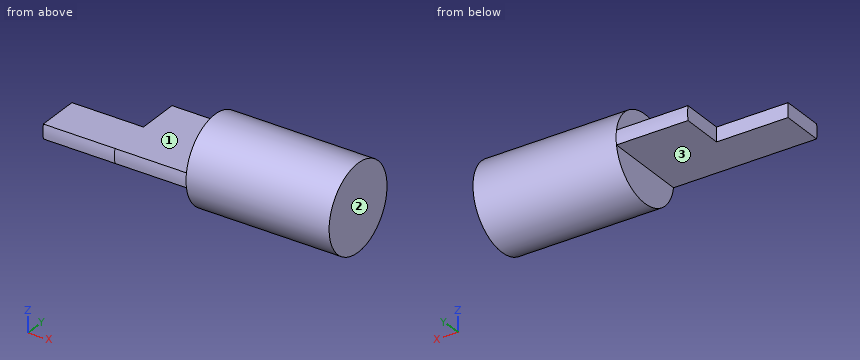
from build123d import *
from build123d.topology import SkipClean

# Parameters (mm, degrees)
SKETCH1_R           = 30
BOSS_EXTRUDE1_DEPTH = 100
BOSS_EXTRUDE2_START = 50
BOSS_EXTRUDE2_DEPTH = 50
BOSS_EXTRUDE3_START = 50
BOSS_EXTRUDE3_DEPTH = 50


with BuildPart() as part:
    # Sketch1 → Boss-Extrude1 (new body)
    with BuildSketch(Plane(origin=(0, 0, 0), x_dir=(0, 0, -1), z_dir=(1, 0, 0))):
        Circle(SKETCH1_R)
    extrude(amount=BOSS_EXTRUDE1_DEPTH)

    # Sketch2 → Boss-Extrude2 (add)
    with SkipClean():  # the faces are left unmerged after this step: merging them gives an invalid solid
        with BuildSketch(Plane.ZY.offset(BOSS_EXTRUDE2_START)):
            with BuildLine():
                Line((5, -29.580398915), (5, 29.580398915))
                ThreePointArc((5, 29.580398915), (0, 30), (-5, 29.580398915))
                Line((-5, 29.580398915), (-5, -29.580398915))
                ThreePointArc((-5, -29.580398915), (0, -30), (5, -29.580398915))
            make_face()
        extrude(amount=-BOSS_EXTRUDE2_DEPTH)

    # Sketch3 → Boss-Extrude3 (add)
    with SkipClean():  # the faces are left unmerged after this step: merging them gives an invalid solid
        with BuildSketch(Plane.ZY.offset(50).offset(BOSS_EXTRUDE3_START)):
            with BuildLine():
                Line((5, 0), (-5, 0))
                Line((-5, 0), (-5, -29.580398915))
                ThreePointArc((-5, -29.580398915), (0, -30), (5, -29.580398915))
                Line((5, -29.580398915), (5, 0))
            make_face()
        extrude(amount=-BOSS_EXTRUDE3_DEPTH)


solid = part.part
Here's how the part is built. I have some questions about the finished solid (model axes, mm). Face numbers are marked on the shaded views. A direction names the side the tool comes from. Round coordinates to 2 decimals unless told otherwise and drop trailing zeros. Loops run counter-clockwise (first coordinate to the right, second up) from the corner with the lowest first, then second, coordinate; pieces in that order, holes last. Notation, with made-up numbers: M 60,-39.5 L 83,-39.5 A7 ccw 83,-34.5 Z; hole C 32.5,60.25 d11. An arc over 180 degrees is marked long. Write each question's results on one line, items separated by ' | '. Start each with the question number.
(1) Will these pins go through, and if not, where does the flat tip stop? P1, Ø6, axis at y = 11.5, z = 5, coming from the -X side; P2, Ø17.5, axis at x = -40, y = 14.5, coming from the -Z side; P3, Ø17.5, axis at x = -62.5, y = -14, coming from the +Z side.
(2) I want a section at C-C (x = 55.5). Please give me the cut outline in (y, z).
(3) I want a section at B-B (y = 23.5). Please give me the cut outline in (x, z), then the cut area to 3 significant figures.
(4) On a 3-axis mill with a long thin cutter (end or side, diameter ignored), from which of +Z, -Z, +X, -X, +Y, -Y can I reach the whole of each face in a straight line? I mean the marked faces 1, 2 and 3. Say none if no direction works.
(5) I want a section at A-A (z = 0). Please give me the cut outline in (x, y).
(6) If I drill on probe 1 along Z at (x, y) = (-6, 18); probe 2 along X at (y, z) = (23, -9.5); probe 3 along Z at (x, y) = (84.5, -11.5), over which ranges is the centre line in solid material (lowest first)? Write a range as from..to.
(7) I want a section at D-D (x = -69). Please give me the cut outline in (y, z).
Solved:
1) P1: stops at x = -50 | P2: stops at z = -5 | P3: stops at z = 5
2) outline: C 0,0 d60
3) outline: M -50,-5 L 0,-5 L 0,-18.65 L 100,-18.65 L 100,18.65 L 0,18.65 L 0,5 L -50,5 Z | area: 4,230 mm²
4) face 1: +Z, -X, +Y, -Y | face 2: +Z, -Z, +X, +Y, -Y | face 3: -Z, -X, +Y, -Y
5) outline: M -100,-30 L 100,-30 L 100,30 L -50,30 L -50,0 L -100,0 Z
6) probe 1: z = -5..5 | probe 2: x = 0..100 | probe 3: z = -27.71..27.71
7) outline: M -29.58,-5 L 0,-5 L 0,5 L -29.58,5 A30 ccw Z
